```python
from build123d import *

# Parameters (mm, degrees)
SKETCH1_W           = 20
SKETCH1_H           = 25
BOSS_EXTRUDE1_DEPTH = 20
SKETCH2_R           = 4
CUT_EXTRUDE1_DEPTH  = 20
SKETCH3_R           = 1.5
CUT_EXTRUDE2_DEPTH  = 21
CUT_EXTRUDE3_DEPTH  = 5


with BuildPart() as part:
    # Sketch1 → Boss-Extrude1 (new body)
    with BuildSketch(Plane(origin=(0, 0, 0), x_dir=(1, 0, 0), z_dir=(0, 1, 0))):
        Rectangle(SKETCH1_W, SKETCH1_H)
    extrude(amount=BOSS_EXTRUDE1_DEPTH)

    # Sketch2 → Cut-Extrude1 (cut)
    with BuildSketch(Plane.XY.offset(12.5)):
        with Locations((0, 10)):
            Circle(SKETCH2_R)
    extrude(amount=-CUT_EXTRUDE1_DEPTH, mode=Mode.SUBTRACT)

    # Sketch3 → Cut-Extrude2 (cut, through all)
    with BuildSketch(Plane(origin=(0, 20, 0), x_dir=(1, 0, 0), z_dir=(0, 1, 0))):
        with Locations((0, 4.5)):
            Circle(SKETCH3_R)
    extrude(amount=-CUT_EXTRUDE2_DEPTH, mode=Mode.SUBTRACT)

    # Sketch4 → Cut-Extrude3 (cut)
    with BuildSketch(Plane(origin=(0, 20, 0), x_dir=(1, 0, 0), z_dir=(0, 1, 0))):
        Polygon((0, 8.6), (-3.550704156, 6.55), (-3.550704156, 2.45), (0, 0.4), (3.550704156, 2.45), (3.550704156, 6.55), align=None)
    extrude(amount=-CUT_EXTRUDE3_DEPTH, mode=Mode.SUBTRACT)


solid = part.part
```
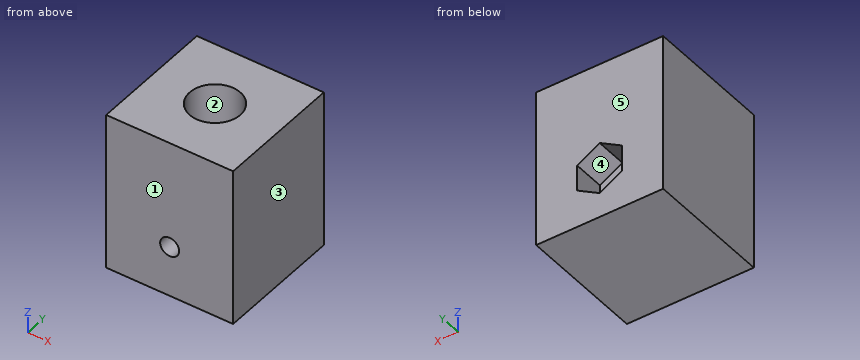
Geometry: final body of the model. Coordinates: model frame, mm. Face numbers are marked on the shaded views. A direction names the side the tool comes from. Round coordinates to 2 decimals unless told otherwise and drop trailing zeros. Order: outer loops, then holes, each group sorted by start corner. A loop starts at its lowest first (then second) coordinate and runs counter-clockwise, first axis right, second up. Notation, with made-up numbers: (55, 11.25) - (110, 11.25) arc R18 ccw to (110, 19.25) - close; hole circle Ø7 at (-24.5, 69.25). An arc over 180 degrees is marked (long way). Write item = value, one per line. Start each with the question number.
Q1. Access query for the marked faces 4 and 5. Directions: +Z, -Z, +X, -X, +Y, -Y. A direction counts if a zero-diameter tool reaches every point of the face in a straight line with its end or side. Return the directions, or none.
Q2. Cut plane D-D on y = 10. Return the cut outline in (x, z).
Q3. Ray query, line 1 (Z direction, x = 0, y = 14.25); line 2 (X direction, y = 14.25, z = -4.5); line 3 (Y direction, x = 0, z = 3.5). Return the intervals inside material, ascending. Write a range as from..to.
Q4. Pin query (flat end, axial travel): pin 1 (2.5 mm diameter, centred on x = 0, z = -4.5, fed in from -Y); pin 2 (4 mm diameter, centred on x = 1, y = 9.5, fed in from +Z); pin 3 (2 mm diameter, centred on x = -1.5, z = -6, fed in from +Y). Return the tip coordinate at first contact, or that it passes through.
Q5. Cut plane B-B on y = 16.5. Return the cut outline in (x, z).
Q6. Pull-direction query (X, two-part tool) for the marked faces 1, 2 and 3; classes: +X half, -X half, draft (parallel to the pull), parting line (faces both ways), or undercut.
Q7. Cut plane C-C on z = 1.5. Return the cut outline in (x, y).
Q8. Cut plane A-A on z = -4.5. Return the cut outline in (x, y).
Outcome:
q1.face_4 = +Y
q1.face_5 = +Z, -Z, +X, -X, +Y
q2.outline = (-10, -12.5) - (10, -12.5) - (10, 12.5) - (4, 12.5) - (4, -7.5) - (-4, -7.5) - (-4, 12.5) - (-10, 12.5) - close
q3.line_1 = -12.5..-6, -3..12.5
q3.line_2 = -10..-1.5, 1.5..10
q3.line_3 = 0..6, 14..20
q4.pin_1 = through
q4.pin_2 = -7.5
q4.pin_3 = 15
q5.outline = (-10, -12.5) - (10, -12.5) - (10, 12.5) - (-10, 12.5) - close; hole (-3.55, -6.55) - (0, -8.6) - (3.55, -6.55) - (3.55, -2.45) - (0, -0.4) - (-3.55, -2.45) - close
q6.face_1 = draft
q6.face_2 = undercut
q6.face_3 = +X half
q7.outline = (-10, 0) - (10, 0) - (10, 20) - (-10, 20) - close; hole circle Ø8 at (0, 10)
q8.outline = (-10, 0) - (-1.5, 0) - (-1.5, 6.29) arc R4 cw to (-1.5, 13.71) - (-1.5, 15) - (-3.55, 15) - (-3.55, 20) - (-10, 20) - close; (1.5, 0) - (10, 0) - (10, 20) - (3.55, 20) - (3.55, 15) - (1.5, 15) - (1.5, 13.71) arc R4 cw to (1.5, 6.29) - close
